Model file for the job. Use its own axes, mm. A direction names the side the tool comes from. Give positions to 0.01 mm unless a question says otherwise; leave off trailing zeros. Write each loop counter-clockwise with the first axis right and the second up, starting at its lowest first coordinate (ties: lowest second). Pieces come first, ordered by that corner, then holes. Notation, with made-up numbers: (44.25, 46) - (63.25, 46) arc R12 cw to (63.25, 65) - close; hole circle Ø11 at (37.5, 15). An arc over 180 degrees is marked (long way). Use a Markdown table: item, result. Add a question column.
```python
from build123d import *

# Parameters (mm, degrees)
BOSS_EXTRUDE1_DEPTH = 0.9
SKETCH2_W           = 9.5
SKETCH2_H           = 7.93
BOSS_EXTRUDE2_DEPTH = 1.6
SKETCH3_R           = 3.1
BOSS_EXTRUDE3_DEPTH = 11.5
SKETCH4_W           = 2
SKETCH4_H           = 19.64
BOSS_EXTRUDE4_DEPTH = 2.15
SKETCH5_W           = 13.5
SKETCH5_H           = 19.3
BOSS_EXTRUDE5_DEPTH = 0.8
SKETCH6_W           = 12.288283072
SKETCH6_H           = 15.069258514
BOSS_EXTRUDE6_DEPTH = 0.8


with BuildPart() as part:
    # Sketch1 → Boss-Extrude1 (new body)
    with BuildSketch(Plane(origin=(0, 0, 0), x_dir=(1, 0, 0), z_dir=(0, 1, 0))):
        Polygon((-12.2, 10.5), (-12.2, -10.5), (12.2, -10.5), (12.2, 10.5), (4.75, 17), (-4.75, 17), align=None)
    extrude(amount=BOSS_EXTRUDE1_DEPTH)

    # Sketch2 → Boss-Extrude2 (add)
    with BuildSketch(Plane(origin=(0, 0, -17), x_dir=(-1, 0, 0), z_dir=(0, 0, -1))):
        with Locations((0, 0.9)):
            Rectangle(SKETCH2_W, SKETCH2_H)
    extrude(amount=BOSS_EXTRUDE2_DEPTH)

    # Sketch3 → Boss-Extrude3 (add)
    with BuildSketch(Plane(origin=(0, 0, -18.6), x_dir=(-1, 0, 0), z_dir=(0, 0, -1))):
        with Locations((0, 0.9)):
            Circle(SKETCH3_R)
    extrude(amount=BOSS_EXTRUDE3_DEPTH)

    # Sketch4 → Boss-Extrude4 (add)
    with BuildSketch(Plane.XZ):
        with Locations((-11, -0.22)):
            Rectangle(SKETCH4_W, SKETCH4_H)
    boss_extrude4 = extrude(amount=BOSS_EXTRUDE4_DEPTH)

    # Mirror1: Boss-Extrude4 across plane
    add(boss_extrude4.mirror(Plane(origin=(0, 0, 0), x_dir=(0, 0, 1), z_dir=(1, 0, 0))))

    # Sketch5 → Boss-Extrude5 (add)
    with BuildSketch(Plane.XZ):
        with Locations((0, 0.137773352)):
            Rectangle(SKETCH5_W, SKETCH5_H)
    extrude(amount=BOSS_EXTRUDE5_DEPTH)

    # Sketch6 → Boss-Extrude6 (add)
    with BuildSketch(Plane.XZ.offset(0.8)):
        with Locations((0, 1.584615241)):
            Rectangle(SKETCH6_W, SKETCH6_H)
    extrude(amount=BOSS_EXTRUDE6_DEPTH)


solid = part.part
```
(1) Band-saw the part on B-B (z = 1). Write the cut outline in (x, y), then the cut area to 3 significant figures.
(2) Band-saw the part on A-A (x = 0). Write the cut outline in (y, z) (3 decimals).
(3) Two-plate mould, pull along Z, no slides. Class faces 5 (the flat face through (-0.2, 0.4, 10.5)), 6 (the flat face through (-10, -1, 0)), 7 (the flat face through (0.5, -0.8, -6.3)): +Z half, -Z half, draft (parallel to the pull), parting line (faces both ways), or undercut.
(4) Flat gauge pins, fed straight in: pin 1 (4.5 mm diameter, centred on x = -1, y = 3, fed in from +Z); pin 2 (0.6 mm diameter, centred on x = 10.5, z = 3.5, fed in from -Y); pin 3 (1.1 mm diameter, centred on y = -1.5, z = 1, fed in from +X); pin 4 (1.5 mm diameter, centred on x = 0, y = -1, fed in from +Z). Where does each tip first touch, or does it go through?
(5) Band-saw the part on D-D (z = -22.5). Write the cut outline in (x, y).
(6) Probe probe 1 along X at (y, z) = (-0.75, 9); probe 2 along Z at (x, y) = (-3, -1); probe 3 along Y at (x, z) = (-9, -3). List the from-to ranges inside material, lowest first. Write a range as [from, to].
(7) Which spindle directions (+Z, -Z, +X, -X, +Y, -Y) get a long thin tool onto all of the face, cutting with end or side? Do faces 1 (the flat face through (0, 0.9, -3)), 2 (the flat face through (0, -1.6, 2)), 3 (the cylindrical face through (-1.43, -1.85, -24.27)), 4 (the flat face through (-12, -1, 0)). Say none if no direction does.
(8) Band-saw the part on C-C (x = -5.75). Write the cut outline in (y, z), then the cut area to 3 significant figures.
Model answer:
| question | item | result |
|---|---|---|
| 1 | outline | (-12.2, 0) - (-12, 0) - (-12, -2.15) - (-10, -2.15) - (-10, 0) - (-6.75, 0) - (-6.75, -0.8) - (-6.14, -0.8) - (-6.14, -1.6) - (6.14, -1.6) - (6.14, -0.8) - (6.75, -0.8) - (6.75, 0) - (10, 0) - (10, -2.15) - (12, -2.15) - (12, 0) - (12.2, 0) - (12.2, 0.9) - (-12.2, 0.9) - close |
| 1 | area | 51.2 mm^2 |
| 2 | outline | (-3.065, -18.6) - (-2.2, -18.6) - (-2.2, -30.1) - (4, -30.1) - (4, -18.6) - (4.865, -18.6) - (4.865, -17) - (0.9, -17) - (0.9, 10.5) - (0, 10.5) - (0, 9.788) - (-0.8, 9.788) - (-0.8, 9.119) - (-1.6, 9.119) - (-1.6, -5.95) - (-0.8, -5.95) - (-0.8, -9.512) - (0, -9.512) - (0, -17) - (-3.065, -17) - close |
| 3 | face 5 | +Z half |
| 3 | face 6 | draft |
| 3 | face 7 | undercut |
| 4 | pin 1 | stops at z = 10.5 |
| 4 | pin 2 | stops at y = -2.15 |
| 4 | pin 3 | stops at x = 12 |
| 4 | pin 4 | stops at z = 9.79 |
| 5 | outline | circle Ø6.2 at (0, 0.9) |
| 6 | probe 1 | x = [-12, -10], [-6.75, 6.75], [10, 12] |
| 6 | probe 2 | z = [-18.6, -17], [-5.95, 9.12] |
| 6 | probe 3 | y = [0, 0.9] |
| 7 | face 1 | +Z, +X, -X, +Y |
| 7 | face 2 | +Z, -Y |
| 7 | face 3 | -Z |
| 7 | face 4 | +Z, -Z, -X, -Y |
| 8 | outline | (-1.6, -5.95) - (-0.8, -5.95) - (-0.8, -9.51) - (0, -9.51) - (0, -16.13) - (0.9, -16.13) - (0.9, 10.5) - (0, 10.5) - (0, 9.79) - (-0.8, 9.79) - (-0.8, 9.12) - (-1.6, 9.12) - close |
| 8 | area | 51.5 mm^2 |
